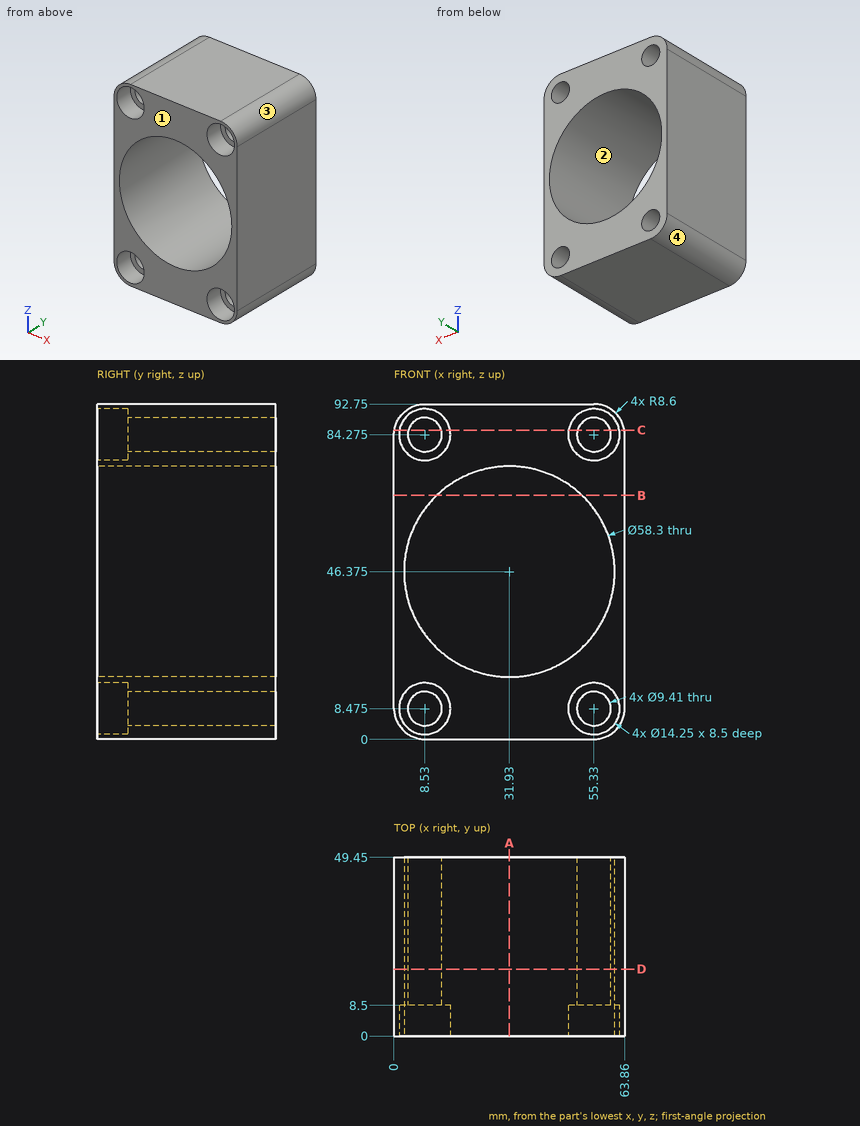
Part print with two shaded views. Sizes in mm from the minimum x, y, z corner. Give positions to 0.01 mm unless a question says otherwise; leave off trailing zeros. Order: outer loops, then holes, each group sorted by start corner. A loop starts at its lowest first (then second) coordinate and runs counter-clockwise, first axis right, second up. Notation, with made-up numbers: M 68,-40 L 83,-40 A33 cw 83,-6 Z; hole C 74,46.5 d3. An arc over 180 degrees is marked long. Use one line per item in the form item = value.
1) Saw through at D-D (y = 18.5). Give the cut face in (x, z) (3 decimals).
Calculated:
outline = M 0,8.6 A8.6 ccw 8.6,0 L 55.26,0 A8.6 ccw 63.86,8.6 L 63.86,84.15 A8.6 ccw 55.26,92.75 L 8.6,92.75 A8.6 ccw 0,84.15 Z; hole C 31.93,46.375 d58.3; hole C 8.53,8.475 d9.41; hole C 8.53,84.275 d9.41; hole C 55.33,8.475 d9.41; hole C 55.33,84.275 d9.41
2) Two-plate mould, pull along Z, no slides. Class the marked faces 1, 2, 3 and 4: released by +Z, released by -Z, zero draft, split by the parting line, or undercut.
Calculated:
face_1 = zero draft
face_2 = undercut
face_3 = released by +Z
face_4 = released by -Z
3) Drop a flat-ended pin along its axis: pin 1 (12 mm diameter, centred on x = 8.53, z = 8.475, fed in from -Y). Give the stop position or say it passes through.
Calculated:
pin_1 = 8.5
4) Saw through at A-A (x = 31.93). Give the cut face in (y, z) (3 decimals), plus the area to 3 significant figures.
Calculated:
outline = M 0,0 L 49.45,0 L 49.45,17.225 L 0,17.225 Z; M 0,75.525 L 49.45,75.525 L 49.45,92.75 L 0,92.75 Z
area = 1,700 mm2
5) Saw through at C-C (z = 85.5). Give the cut face in (x, y), plus the area to 3 significant figures.
Calculated:
outline = M 0.11,0 L 1.51,0 L 1.51,8.5 L 3.99,8.5 L 3.99,49.45 L 0.11,49.45 Z; M 13.07,8.5 L 15.55,8.5 L 15.55,0 L 48.31,0 L 48.31,8.5 L 50.79,8.5 L 50.79,49.45 L 13.07,49.45 Z; M 59.87,8.5 L 62.35,8.5 L 62.35,0 L 63.75,0 L 63.75,49.45 L 59.87,49.45 Z
area = 2,160 mm2
6) Saw through at B-B (z = 67.5). Give the cut face in (x, y).
Calculated:
outline = M 0,0 L 11.84,0 L 11.84,49.45 L 0,49.45 Z; M 52.02,0 L 63.86,0 L 63.86,49.45 L 52.02,49.45 Z
7) Probe probe 1 along X at (y, z) = (20.5, 84); probe 2 along X at (y, z) = (21.5, 24); probe 3 along Z at (x, y) = (8.53, 32.5). List the from-to ranges inside material, lowest first.
Calculated:
probe_1 = 0 to 3.83, 13.23 to 50.63, 60.03 to 63.86
probe_2 = 0 to 13.25, 50.61 to 63.86
probe_3 = 0 to 3.77, 13.18 to 28.99, 63.76 to 79.57, 88.98 to 92.75
